Geometry: final body of the model. Coordinates: model frame, mm. Face numbers are marked on the shaded views. A direction names the side the tool comes from. Give positions to 0.01 mm unless a question says otherwise; leave off trailing zeros. Loops run counter-clockwise (first coordinate to the right, second up) from the corner with the lowest first, then second, coordinate; pieces in that order, holes last.
1. Section C-C, the plane z = -145.5. Output: boundary loops of the cut face in (x, y).
2. Section A-A, the plane x = 0. Output: boundary loops of the cut face in (y, z).
3. Material intervals for line 1 along Z through (x, y) = (-100, -9); line 2 along X through (y, z) = (15, -9.75); line 3 along X through (y, z) = (35, -176), sorted ascending.
4. First-contact query: P1, Ø5, axis at x = -60, y = 30, coming from the -Z side; P2, Ø3.5, axis at x = 60, y = 180, coming from the +Z side; P3, Ø8, axis at y = 134.5, z = -37, coming from the +X side; P4, Ø12, axis at x = 33, y = 156.5, coming from the +Z side. Flat tips, straight axial feed; report the tip coordinate or a pass-through.
5. Section B-B, the plane z = -190. Output: boundary loops of the cut face in (x, y), then the cut area to 3 significant figures.
6. Access query for the marked faces 1, 2 and 3. Directions: +Z, -Z, +X, -X, +Y, -Y. A direction counts if a zero-diameter tool reaches every point of the face in a straight line with its end or side. Return the directions, or none.
7. Draft query along X for the marked faces 4, 5, 6 and 7. Return one class per face: +X half, -X half, draft (parallel to the pull), parting line (faces both ways), or undercut.
8. Section D-D, the plane x = 73.5. Output: boundary loops of the cut face in (y, z), then the cut area to 3 significant figures.
from build123d import *

# Parameters (mm, degrees)
ESBO_O1_W                      = 200
ESBO_O1_H                      = 200
RESSALTO_EXTRUS_O1_DEPTH       = 20
RESSALTO_EXTRUS_O2_DEPTH       = 10
ESBO_O3_W                      = 260
ESBO_O3_H                      = 220
RESSALTO_EXTRUS_O3_DEPTH       = 20
CORTE_EXTRUS_O1_REACH          = 326.5
ESBO_O4_R                      = 11
PADR_O_LINEAR1_COUNT           = 2
PADR_O_LINEAR1_PITCH           = 100
PADR_O_LINEAR1_COL_COUNT       = 2
PADR_O_LINEAR1_COL_PITCH       = 100
PADR_O_LINEAR2_COUNT           = 2
PADR_O_LINEAR2_PITCH           = 140
PADR_O_LINEAR2_COPY_1_REACH    = 326.5
PADR_O_LINEAR2_COPY_1_SKETCH_R = 11
PADR_O_LINEAR2_COPY_2_REACH    = 326.5
PADR_O_LINEAR2_COPY_2_SKETCH_R = 11
PADR_O_LINEAR3_COUNT           = 15
PADR_O_LINEAR3_PITCH           = 15


with BuildPart() as part:
    # Esboço1 → Ressalto-extrusão1 (new body)
    with BuildSketch(Plane.XY):
        with Locations((0, 100)):
            Rectangle(ESBO_O1_W, ESBO_O1_H)
    extrude(amount=-RESSALTO_EXTRUS_O1_DEPTH)

    # Esboço2 → Ressalto-extrusão2 (add, symmetric)
    with BuildSketch(Plane(origin=(60, 0, 0), x_dir=(0, 0, -1), z_dir=(1, 0, 0))):
        Polygon((20, 0), (20, 200), (220, 0), align=None)
    ressalto_extrus_o2 = extrude(amount=RESSALTO_EXTRUS_O2_DEPTH, both=True)

    # Espelhar1: Ressalto-extrusão2 across plane
    add(ressalto_extrus_o2.mirror(Plane(origin=(0, 0, 0), x_dir=(0, 0, 1), z_dir=(1, 0, 0))))

    # Esboço3 → Ressalto-extrusão3 (add)
    with BuildSketch(Plane.XZ):
        with Locations((0, -110)):
            Rectangle(ESBO_O3_W, ESBO_O3_H)
    extrude(amount=RESSALTO_EXTRUS_O3_DEPTH)

    # Esboço4 → Corte-extrusão1 (cut, up to next)
    with BuildSketch(Plane(origin=(0, 0, 0), x_dir=(1, 0, 0), z_dir=(0, 1, 0)), mode=Mode.PRIVATE) as corte_extrus_o1_sk1:
        with Locations(Location((0, 190, 0), (0, 0, 180))):
            Circle(ESBO_O4_R)
    corte_extrus_o1_tool1 = extrude(corte_extrus_o1_sk1.sketch, amount=-CORTE_EXTRUS_O1_REACH, mode=Mode.PRIVATE) & part.part
    corte_extrus_o1 = corte_extrus_o1_tool1.solids().sort_by_distance((0, 0, -190))[0]
    add(corte_extrus_o1, mode=Mode.SUBTRACT)

    # Padrão linear1: Corte-extrusão1 ×2
    with Locations(*[(i * PADR_O_LINEAR1_PITCH, 0, 0) for i in range(1, PADR_O_LINEAR1_COUNT)]):
        add(corte_extrus_o1, mode=Mode.SUBTRACT)

    # Padrão linear1 col: Corte-extrusão1 ×2
    with Locations(*[(-i * PADR_O_LINEAR1_COL_PITCH, 0, 0) for i in range(1, PADR_O_LINEAR1_COL_COUNT)]):
        add(corte_extrus_o1, mode=Mode.SUBTRACT)

    # Padrão linear2: Corte-extrusão1 ×2
    with Locations(*[(0, 0, i * PADR_O_LINEAR2_PITCH) for i in range(1, PADR_O_LINEAR2_COUNT)]):
        add(corte_extrus_o1, mode=Mode.SUBTRACT)

    # Padrão linear2 copy 1 sketch → Padrão linear2 copy 1 (cut, up to next)
    with BuildSketch(Plane(origin=(100, 0, 140), x_dir=(1, 0, 0), z_dir=(0, 1, 0)), mode=Mode.PRIVATE) as padr_o_linear2_copy_1_sk1:
        with Locations(Location((0, 190, 0), (0, 0, 180))):
            Circle(PADR_O_LINEAR2_COPY_1_SKETCH_R)
    padr_o_linear2_copy_1_tool1 = extrude(padr_o_linear2_copy_1_sk1.sketch, amount=-PADR_O_LINEAR2_COPY_1_REACH, mode=Mode.PRIVATE) & part.part
    add(padr_o_linear2_copy_1_tool1.solids().sort_by_distance((100, 0, -50))[0], mode=Mode.SUBTRACT)

    # Padrão linear2 copy 2 sketch → Padrão linear2 copy 2 (cut, up to next)
    with BuildSketch(Plane(origin=(-100, 0, 140), x_dir=(1, 0, 0), z_dir=(0, 1, 0)), mode=Mode.PRIVATE) as padr_o_linear2_copy_2_sk1:
        with Locations(Location((0, 190, 0), (0, 0, 180))):
            Circle(PADR_O_LINEAR2_COPY_2_SKETCH_R)
    padr_o_linear2_copy_2_tool1 = extrude(padr_o_linear2_copy_2_sk1.sketch, amount=-PADR_O_LINEAR2_COPY_2_REACH, mode=Mode.PRIVATE) & part.part
    add(padr_o_linear2_copy_2_tool1.solids().sort_by_distance((-100, 0, -50))[0], mode=Mode.SUBTRACT)

    # Esboço7 → Furo roscado de M51 (revolve, cut)
    with BuildSketch(Plane(origin=(-60, -15, 0), x_dir=(0, -1, 0), z_dir=(1, 0, 0))):
        Polygon((0, 0), (0, 28.2618073), (2.1, 27), (2.1, 0.425), (2.525, 0), align=None)
    furo_roscado_de_m51 = revolve(axis=Axis((-60, -15, 6.35), (0, 0, -1)), mode=Mode.SUBTRACT)

    # Padrão linear3: Furo roscado de M51 ×15
    with Locations(*[(0, i * PADR_O_LINEAR3_PITCH, 0) for i in range(1, PADR_O_LINEAR3_COUNT)]):
        add(furo_roscado_de_m51, mode=Mode.SUBTRACT)

    # Espelhar2: Furo roscado de M51 across plane
    add(furo_roscado_de_m51.mirror(Plane(origin=(0, 0, 0), x_dir=(0, 0, 1), z_dir=(1, 0, 0))), mode=Mode.SUBTRACT)

    # Espelhar2 copy 1 sketch → Espelhar2 copy 1 (revolve, cut)
    with BuildSketch(Plane(origin=(60, 0, 0), x_dir=(0, -1, 0), z_dir=(-1, 0, 0))):
        Polygon((0, 0), (0, -28.2618073), (2.1, -27), (2.1, -0.425), (2.525, 0), align=None)
    revolve(axis=Axis((60, 0, 6.35), (0, 0, 1)), mode=Mode.SUBTRACT)

    # Espelhar2 copy 2 sketch → Espelhar2 copy 2 (revolve, cut)
    with BuildSketch(Plane(origin=(60, 15, 0), x_dir=(0, -1, 0), z_dir=(-1, 0, 0))):
        Polygon((0, 0), (0, -28.2618073), (2.1, -27), (2.1, -0.425), (2.525, 0), align=None)
    revolve(axis=Axis((60, 15, 6.35), (0, 0, 1)), mode=Mode.SUBTRACT)

    # Espelhar2 copy 3 sketch → Espelhar2 copy 3 (revolve, cut)
    with BuildSketch(Plane(origin=(60, 30, 0), x_dir=(0, -1, 0), z_dir=(-1, 0, 0))):
        Polygon((0, 0), (0, -28.2618073), (2.1, -27), (2.1, -0.425), (2.525, 0), align=None)
    revolve(axis=Axis((60, 30, 6.35), (0, 0, 1)), mode=Mode.SUBTRACT)

    # Espelhar2 copy 4 sketch → Espelhar2 copy 4 (revolve, cut)
    with BuildSketch(Plane(origin=(60, 45, 0), x_dir=(0, -1, 0), z_dir=(-1, 0, 0))):
        Polygon((0, 0), (0, -28.2618073), (2.1, -27), (2.1, -0.425), (2.525, 0), align=None)
    revolve(axis=Axis((60, 45, 6.35), (0, 0, 1)), mode=Mode.SUBTRACT)

    # Espelhar2 copy 5 sketch → Espelhar2 copy 5 (revolve, cut)
    with BuildSketch(Plane(origin=(60, 60, 0), x_dir=(0, -1, 0), z_dir=(-1, 0, 0))):
        Polygon((0, 0), (0, -28.2618073), (2.1, -27), (2.1, -0.425), (2.525, 0), align=None)
    revolve(axis=Axis((60, 60, 6.35), (0, 0, 1)), mode=Mode.SUBTRACT)

    # Espelhar2 copy 6 sketch → Espelhar2 copy 6 (revolve, cut)
    with BuildSketch(Plane(origin=(60, 75, 0), x_dir=(0, -1, 0), z_dir=(-1, 0, 0))):
        Polygon((0, 0), (0, -28.2618073), (2.1, -27), (2.1, -0.425), (2.525, 0), align=None)
    revolve(axis=Axis((60, 75, 6.35), (0, 0, 1)), mode=Mode.SUBTRACT)

    # Espelhar2 copy 7 sketch → Espelhar2 copy 7 (revolve, cut)
    with BuildSketch(Plane(origin=(60, 90, 0), x_dir=(0, -1, 0), z_dir=(-1, 0, 0))):
        Polygon((0, 0), (0, -28.2618073), (2.1, -27), (2.1, -0.425), (2.525, 0), align=None)
    revolve(axis=Axis((60, 90, 6.35), (0, 0, 1)), mode=Mode.SUBTRACT)

    # Espelhar2 copy 8 sketch → Espelhar2 copy 8 (revolve, cut)
    with BuildSketch(Plane(origin=(60, 105, 0), x_dir=(0, -1, 0), z_dir=(-1, 0, 0))):
        Polygon((0, 0), (0, -28.2618073), (2.1, -27), (2.1, -0.425), (2.525, 0), align=None)
    revolve(axis=Axis((60, 105, 6.35), (0, 0, 1)), mode=Mode.SUBTRACT)

    # Espelhar2 copy 9 sketch → Espelhar2 copy 9 (revolve, cut)
    with BuildSketch(Plane(origin=(60, 120, 0), x_dir=(0, -1, 0), z_dir=(-1, 0, 0))):
        Polygon((0, 0), (0, -28.2618073), (2.1, -27), (2.1, -0.425), (2.525, 0), align=None)
    revolve(axis=Axis((60, 120, 6.35), (0, 0, 1)), mode=Mode.SUBTRACT)

    # Espelhar2 copy 10 sketch → Espelhar2 copy 10 (revolve, cut)
    with BuildSketch(Plane(origin=(60, 135, 0), x_dir=(0, -1, 0), z_dir=(-1, 0, 0))):
        Polygon((0, 0), (0, -28.2618073), (2.1, -27), (2.1, -0.425), (2.525, 0), align=None)
    revolve(axis=Axis((60, 135, 6.35), (0, 0, 1)), mode=Mode.SUBTRACT)

    # Espelhar2 copy 11 sketch → Espelhar2 copy 11 (revolve, cut)
    with BuildSketch(Plane(origin=(60, 150, 0), x_dir=(0, -1, 0), z_dir=(-1, 0, 0))):
        Polygon((0, 0), (0, -28.2618073), (2.1, -27), (2.1, -0.425), (2.525, 0), align=None)
    revolve(axis=Axis((60, 150, 6.35), (0, 0, 1)), mode=Mode.SUBTRACT)

    # Espelhar2 copy 12 sketch → Espelhar2 copy 12 (revolve, cut)
    with BuildSketch(Plane(origin=(60, 165, 0), x_dir=(0, -1, 0), z_dir=(-1, 0, 0))):
        Polygon((0, 0), (0, -28.2618073), (2.1, -27), (2.1, -0.425), (2.525, 0), align=None)
    revolve(axis=Axis((60, 165, 6.35), (0, 0, 1)), mode=Mode.SUBTRACT)

    # Espelhar2 copy 13 sketch → Espelhar2 copy 13 (revolve, cut)
    with BuildSketch(Plane(origin=(60, 180, 0), x_dir=(0, -1, 0), z_dir=(-1, 0, 0))):
        Polygon((0, 0), (0, -28.2618073), (2.1, -27), (2.1, -0.425), (2.525, 0), align=None)
    revolve(axis=Axis((60, 180, 6.35), (0, 0, 1)), mode=Mode.SUBTRACT)

    # Espelhar2 copy 14 sketch → Espelhar2 copy 14 (revolve, cut)
    with BuildSketch(Plane(origin=(60, 195, 0), x_dir=(0, -1, 0), z_dir=(-1, 0, 0))):
        Polygon((0, 0), (0, -28.2618073), (2.1, -27), (2.1, -0.425), (2.525, 0), align=None)
    revolve(axis=Axis((60, 195, 6.35), (0, 0, 1)), mode=Mode.SUBTRACT)


solid = part.part
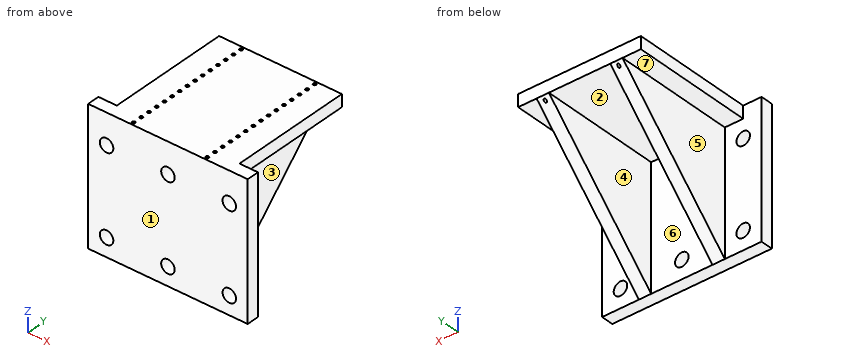
Answers below:
1. outline: (-130, -20) - (130, -20) - (130, 0) - (70, 0) - (70, 74.5) - (50, 74.5) - (50, 0) - (-50, 0) - (-50, 74.5) - (-70, 74.5) - (-70, 0) - (-130, 0) - close
2. outline: (-20, -220) - (0, -220) - (0, -201) - (-20, -201) - close; (-20, -179) - (0, -179) - (0, -61) - (-20, -61) - close; (-20, -39) - (0, -39) - (0, -20) - (200, -20) - (200, 0) - (-20, 0) - close
3. line 1: z = -220 to -201, -179 to -61, -39 to 0
3. line 2: x = -100 to -62.1, -57.9 to 57.9, 62.1 to 100
3. line 3: x = -70 to -50, 50 to 70
4. P1: stops at z = -192.5
4. P2: stops at z = -27.21
4. P3: stops at x = 70
4. P4: stops at z = 0
5. outline: (-130, -20) - (-111, -20) - (-111, 0) - (-130, 0) - close; (-89, -20) - (-11, -20) - (-11, 0) - (-50, 0) - (-50, 30) - (-70, 30) - (-70, 0) - (-89, 0) - close; (11, -20) - (89, -20) - (89, 0) - (70, 0) - (70, 30) - (50, 30) - (50, 0) - (11, 0) - close; (111, -20) - (130, -20) - (130, 0) - (111, 0) - close
5. area: 5,080 mm2
6. face 1: +Z, -Z, +X, -X, -Y
6. face 2: -Z, +Y
6. face 3: -Z, +X, +Y
7. face 4: undercut
7. face 5: -X half
7. face 6: undercut
7. face 7: draft
8. outline: (-20, -220) - (0, -220) - (0, -20) - (200, -20) - (200, 0) - (-20, 0) - close
8. area: 8,400 mm2
